from build123d import *

# Parameters (mm, degrees)
F0_R      = 12.7
F1_DEPTH  = 76.2
F1_FACE_R = 12.7
F2_DEPTH  = 25.4
F2_TAPER  = 30
F3_R      = 50.8
F4_T      = -2.54
F6_DEPTH  = 1.27
F7_COUNT  = 10


with BuildPart() as f1:
    # F0 (on Top) → F1 (new body)
    with BuildSketch(Plane.XY):
        Circle(F0_R)
    extrude(amount=F1_DEPTH)

    # F1_face (on face) → F2 (join)
    with BuildSketch(Plane.XY.offset(76.2)):
        Circle(F1_FACE_R)
    extrude(amount=F2_DEPTH, taper=F2_TAPER)

    # F3
    f3_edges = [f1.edges().sort_by_distance(p)[0] for p in [
        (-12.7, 0, 76.2),
    ]]
    fillet(f3_edges, radius=F3_R)

    # F4
    f4_openings = [f1.faces().sort_by_distance(p)[0] for p in [
        (0, 0, 0),
    ]]
    offset(amount=F4_T, openings=f4_openings)

    # F5 (on Front) → F6 (join, symmetric)
    with BuildSketch(Plane.XZ):
        Polygon((-35.56, 0), (-10.16, 0), (-10.16, 25.4), align=None)
    extrude(amount=F6_DEPTH, both=True)

    # F7: F1 ×10 about axis
    f7_axis = Axis((0, 0, 0), (0, 0, 1))


with BuildPart() as f1_1:
    add(f1.part)
    for i in range(1, F7_COUNT):
        add(f1.part.rotate(f7_axis, i * 360 / F7_COUNT))


solid = f1_1.part
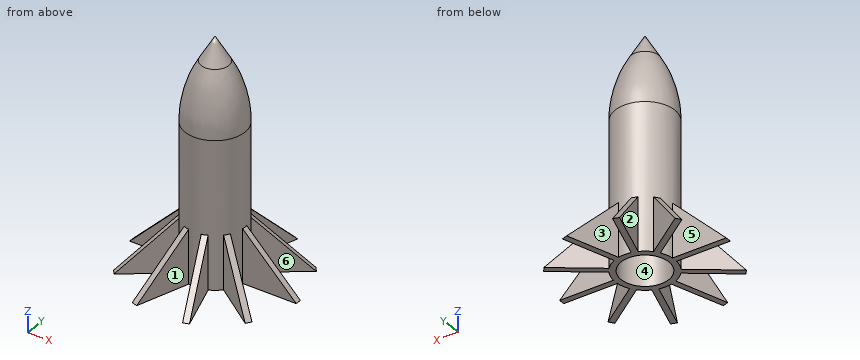
Build history of the part. All positions in model axes, mm. Face numbers are marked on the shaded views. A direction names the side the tool comes from. Round coordinates to 2 decimals unless told otherwise and drop trailing zeros. Loops run counter-clockwise (first coordinate to the right, second up) from the corner with the lowest first, then second, coordinate; pieces in that order, holes last. Notation, with made-up numbers: (65.5, 28.5) -> (105.5, 28.5) arc R9 cw to (105.5, 42.5) -> close; hole circle Ø8 at (75, 43.25). An arc over 180 degrees is marked (long way). One line per item, written item: value. Start each with the question number.
Q1. 3-axis set-ups, long thin cutter, end or side, ignore diameter. For the marked faces 1, 2 and 3: which of +Z, -Z, +X, -X, +Y, -Y reach the whole face in a straight line?
Q2. Probe line 1 along Y through (x, z) = (0, 34); line 2 along X through (y, z) = (9, 28.5). List the from-to ranges inside material, lowest first.
Q3. Cut at B-B on z = 49. List the corners of the cut face in (x, y).
Q4. Drop flat-ended pins along their axis: pin 1 Ø7 at (x, z) = (20, 15.5) entering from -Y; pin 2 Ø4 at (y, z) = (-1.5, 71.5) entering from +X; pin 3 Ø4 at (x, z) = (-6.5, 51) entering from -Y. Give the stop position or say it passes through.
Q5. Two-plate mould, pull along X, no slides. Class the marked faces 4, 5 and 6: released by +X, released by -X, zero draft, split by the parting line, or undercut.
Q6. Cut at A-A on y = 15.5. List the corners of the cut face in (x, z).
Computed:
1. face 1: +Z, -Z, -Y
1. face 2: +Z, -Z
1. face 3: +Z, -Z, +Y
2. line 1: -12.7 to -10.16, 10.16 to 12.7
2. line 2: -8.96 to -4.71, 4.71 to 8.96
3. outline: circle Ø25.4 at (0, 0); hole circle Ø20.32 at (0, 0)
4. pin 1: y = -14.26
4. pin 2: x = 12.18
4. pin 3: y = -11.88
5. face 4: undercut
5. face 5: zero draft
5. face 6: released by +X
6. outline: (-23.49, 0) -> (-19.17, 0) -> (-19.17, 10.94) -> (-23.49, 7.44) -> close; (-6.37, 0) -> (-3.7, 0) -> (-3.7, 19.67) -> (-6.37, 18.85) -> close; (3.7, 0) -> (6.37, 0) -> (6.37, 18.85) -> (3.7, 19.67) -> close; (19.17, 0) -> (23.49, 0) -> (23.49, 7.44) -> (19.17, 10.94) -> close
